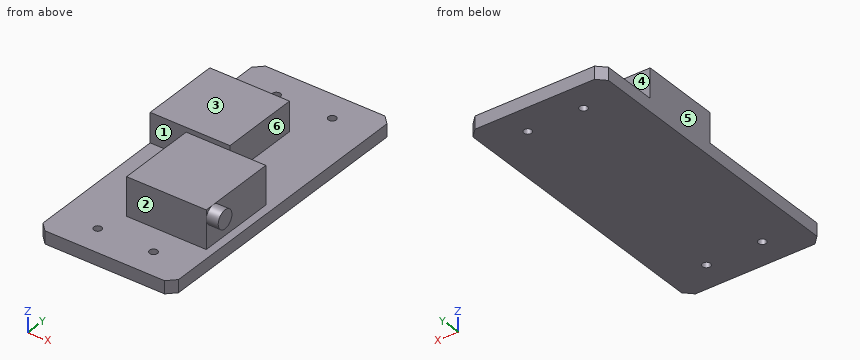
Autodesk Fusion 360 part; units mm, degrees
sketch "Skizze1" plane through (0, 0, 0) normal (0, 0, 1) x (1, 0, 0)
  line L0 (2.5, 0) -> (15.28, 0)
  line L1 (17.78, 2.5) -> (17.78, 16.55)
  line L2 (15.28, 19.05) -> (2.5, 19.05)
  line L3 (0, 16.55) -> (0, 2.5)
  arc A0 (2.5, 19.05) -> (0, 16.55) centre (2.5, 16.55) ccw
  arc A1 (17.78, 16.55) -> (15.28, 19.05) centre (15.28, 16.55) ccw
  arc A2 (15.28, 0) -> (17.78, 2.5) centre (15.28, 2.5) ccw
  arc A3 (0, 2.5) -> (2.5, 0) centre (2.5, 2.5) ccw
  circle A4 centre (2.5, 16.55) radius 1
  circle A5 centre (15.2, 16.55) radius 1
  circle A6 centre (0.89, 2.5) radius 0.5
  circle A7 centre (3.5567, 2.5) radius 0.5
  circle A8 centre (6.2233, 2.5) radius 0.5
  circle A9 centre (8.89, 2.5) radius 0.5
  circle A10 centre (11.5567, 2.5) radius 0.5
  circle A11 centre (14.2233, 2.5) radius 0.5
  circle A12 centre (16.89, 2.5) radius 0.5
  point P0 (17.78, 0)
  dimension "d3" = 17.78
  dimension "d4" = 19.05
  dimension "d5" = 2.5
  dimension "d6" = 2
  dimension "d9" = 12.7
  dimension "d10" = 0
  dimension "d11" = 1
  dimension "d12" = 2.5
  dimension "d15" = 16
  dimension "d16" = 0
  dimension "d17" = 8.89
extrude "Extrusion1" add sketch "Skizze1" along normal blind 1.6

Autodesk Fusion 360 part; units mm, degrees
sketch "Skizze1" plane through (0, 0, 0) normal (0, 0, 1) x (1, 0, 0)
  line L0 (1, 0) -> (16, 0)
  line L1 (17, 1) -> (17, 36)
  line L2 (16, 37) -> (1, 37)
  line L3 (0, 36) -> (0, 1)
  circle A0 centre (5, 33.5) radius 0.5
  circle A1 centre (12, 33.5) radius 0.5
  circle A2 centre (5, 3.5) radius 0.5
  circle A3 centre (12, 3.5) radius 0.5
  line L4 (0, 29) -> (10, 29)
  line L5 (10, 29) -> (10, 19)
  line L6 (10, 19) -> (0, 19)
  line L7 (0, 19) -> (0, 29)
  line L8 (16, 7) -> (6, 7)
  line L9 (6, 7) -> (6, 17)
  line L10 (6, 17) -> (16, 17)
  line L11 (16, 17) -> (16, 7)
  line L12 (1, 37) -> (0, 36)
  line L13 (17, 36) -> (16, 37)
  line L14 (1, 0) -> (0, 1)
  line L15 (16, 0) -> (17, 1)
  point P0 (17, 0)
  point P1 (17, 37)
  point P2 (0, 37)
  dimension "d1" = 17
  dimension "d2" = 37
  dimension "d3" = 1
  dimension "d4" = 5
  dimension "d5" = 3.5
  dimension "d8" = 7
  dimension "d9" = -30
  dimension "d10" = 10
  dimension "d11" = 10
  dimension "d12" = 8
  dimension "d13" = 10
  dimension "d14" = 10
  dimension "d15" = 7
  dimension "d16" = 1
  dimension "d28" = 1
  dimension "d29" = 1
  dimension "d30" = 1
  dimension "d31" = 1
  dimension "d32" = 1
  dimension "d33" = 1
  dimension "d34" = 1
  dimension "d35" = 1
extrude "Extrusion1" add sketch "Skizze1" along normal blind 1.6 contours L0 L1 L2 L3 L4 L5 L6 L12 L13 L14 L15
extrude "Extrusion2" add sketch "Skizze1" along normal blind 5.3 contours L3 L4 L5 L6 L7
extrude "Extrusion3" add sketch "Skizze1" along normal blind 6.4 contours L8 L9 L10 L11
sketch "Skizze2" plane through (16, 0, 0) normal (1, 0, 0) x (0, 1, 0)
  line L0 (17, 1.6) -> (17, 6.4)
  line L1 (17, 6.4) -> (7, 6.4)
  line L2 (7, 6.4) -> (7, 1.6)
  circle A0 centre (8.15, 5.25) radius 1.15
  line L3 (7, 1.6) -> (17, 1.6)
  dimension "d23" = 2.3
  dimension "d24" = 1.15
  dimension "d25" = 1.15
extrude "Extrusion4" add sketch "Skizze2" along normal blind 1.5 contours A0
equation "d29 = d28"
equation "d31 = d30"
equation "d33 = d32"
equation "d35 = d34"
Source: CAD feature listing. Evaluate the final solid. Frame: model axes, mm. Face numbers are marked on the shaded views. A direction names the side the tool comes from. Give positions to 0.01 mm unless a question says otherwise; leave off trailing zeros. Loops run counter-clockwise (first coordinate to the right, second up) from the corner with the lowest first, then second, coordinate; pieces in that order, holes last. Notation, with made-up numbers: (51, 32) -> (72, 32) arc R17 cw to (72, 39) -> close; hole circle Ø9 at (-38, -35.75). An arc over 180 degrees is marked (long way). Use a Markdown table: item, result. Add a question column.
(1) Section query A-A (x = 12). Output: boundary loops of the cut face in (y, z).
(2) Section query C-C (y = 33.5). Output: boundary loops of the cut face in (x, z).
(3) Section query D-D (y = 13.5). Output: boundary loops of the cut face in (x, z).
(4) Pull-direction query (Y, two-part tool) for the marked faces 1, 2 and 3; classes: +Y half, -Y half, draft (parallel to the pull), parting line (faces both ways), or undercut.
(5) Access query for the marked faces 4, 5 and 6. Directions: +Z, -Z, +X, -X, +Y, -Y. A direction counts if a zero-diameter tool reaches every point of the face in a straight line with its end or side. Return the directions, or none.
(6) Ray query, line 1 (Y direction, x = 12, z = 0.4); line 2 (X direction, y = 33.5, z = 0.45); line 3 (Y direction, x = 7.25, z = 4.75). Return the intervals inside material, ascending.
(7) Section query B-B (z = 2.75). Output: boundary loops of the cut face in (x, y), then the cut area to 3 significant figures.
(8) First-contact query: pin 1 Ø1.4 at (y, z) = (13.5, 5) entering from +X; pin 2 Ø1.8 at (y, z) = (10.5, 0.5) entering from +X; pin 3 Ø2.5 at (y, z) = (14, 4.5) entering from -X. Flat tips, straight axial feed; report the tip coordinate or a pass-through.
Checked values:
| question | item | result |
|---|---|---|
| 1 | outline | (0, 0) -> (3, 0) -> (3, 1.6) -> (0, 1.6) -> close; (4, 0) -> (33, 0) -> (33, 1.6) -> (17, 1.6) -> (17, 6.4) -> (7, 6.4) -> (7, 1.6) -> (4, 1.6) -> close; (34, 0) -> (37, 0) -> (37, 1.6) -> (34, 1.6) -> close |
| 2 | outline | (0, 0) -> (4.5, 0) -> (4.5, 1.6) -> (0, 1.6) -> close; (5.5, 0) -> (11.5, 0) -> (11.5, 1.6) -> (5.5, 1.6) -> close; (12.5, 0) -> (17, 0) -> (17, 1.6) -> (12.5, 1.6) -> close |
| 3 | outline | (0, 0) -> (17, 0) -> (17, 1.6) -> (16, 1.6) -> (16, 6.4) -> (6, 6.4) -> (6, 1.6) -> (0, 1.6) -> close |
| 4 | face 1 | undercut |
| 4 | face 2 | -Y half |
| 4 | face 3 | draft |
| 5 | face 4 | +Z, +X, -X, +Y |
| 5 | face 5 | +Z, -Z, -X, +Y, -Y |
| 5 | face 6 | +Z, +X, +Y |
| 6 | line 1 | 0 to 3, 4 to 33, 34 to 37 |
| 6 | line 2 | 0 to 4.5, 5.5 to 11.5, 12.5 to 17 |
| 6 | line 3 | 7 to 17, 19 to 29 |
| 7 | outline | (0, 19) -> (10, 19) -> (10, 29) -> (0, 29) -> close; (6, 7) -> (16, 7) -> (16, 17) -> (6, 17) -> close |
| 7 | area | 200 mm^2 |
| 8 | pin 1 | x = 16 |
| 8 | pin 2 | x = 17 |
| 8 | pin 3 | x = 6 |
